Autodesk Inventor part; units mm, degrees
ref_plane "Arbeitsebene1" through (0, 0, 1.46) normal (0, 0, -1) x (-1, 0, 0)
ref_plane "Arbeitsebene2" through (-0.6, -3.21, 0) normal (0, -1, 0) x (1, 0, 0)
ref_plane "YZ Plane" through (0, 0, 0) normal (1, 0, 0) x (0, 1, 0)
sketch "Skizze2" plane through (0, 0, 0) normal (0, 0, 1) x (1, 0, 0)
  line L0 (0, 0) -> (-0.6, 0)
  line L1 (-0.6, 0) -> (-0.6, 0.6)
  line L2 (-0.6, 0.6) -> (0, 0.6)
  line L3 (0, 0.6) -> (0, 0)
  dimension "d0" = 0.6
  dimension "d1" = 0.6
extrude "Extrusion1" add sketch "Skizze2" along normal blind 9.46
ref_plane "Arbeitsebene1" through (0, 0, 1.46) normal (0, 0, -1) x (-1, 0, 0)
sketch "Skizze3" plane through (0, 0, 1.46) normal (0, 0, -1) x (-1, 0, 0)
  line L0 (1.57, 1.57) -> (-0.97, 1.57)
  line L1 (-0.97, 1.57) -> (-0.97, -0.97)
  line L2 (-0.97, -0.97) -> (1.57, -0.97)
  line L3 (1.57, -0.97) -> (1.57, 1.57)
  line L4 (0.6, 0) -> (0.6, 0.6)
  line L5 (0, 0.6) -> (0.6, 0.6)
  point P0 (0, 0)
  dimension "d5" = 2.54
  dimension "d6" = 2.54
  dimension "d7" = 0.97
  dimension "d8" = 0.97
extrude "Extrusion2" add sketch "Skizze3" against normal blind 2.5
chamfer "Fase1" distance 0.25 angle 45 4 edges at (0.97, -0.97, 2.71) (-1.57, -0.97, 2.71) (-1.57, 1.57, 2.71) (0.97, 1.57, 2.71)
sketch "Skizze8" plane through (-0.6, 0, 0) normal (0, -1, 0) x (1, 0, 0)
  line L0 (0, 0) -> (0.6, 0)
  line L1 (0, 0) -> (0, 1.46)
  line L2 (0.6, 0) -> (0, 0)
  line L3 (0, 0) -> (0, 0.6)
  line L4 (0, 0.6) -> (0.6, 0.6)
  line L5 (0.6, 0.6) -> (0.6, 0)
  dimension "d33" = 0.6
extrude "Extrusion6" add sketch "Skizze8" along normal blind 3.46
chamfer "Fase3" distance 0.15 angle 45 8 edges at (-0.6, 0.3, 9.46) (-0.3, 0, 9.46) (0, 0.3, 9.46) (-0.3, 0.6, 9.46) (0, -3.46, 0.3) (-0.3, -3.46, 0.6) (-0.3, -3.46, 0) (-0.6, -3.46, 0.3)
ref_plane "Arbeitsebene2" through (-0.6, -3.21, 0) normal (0, -1, 0) x (1, 0, 0)
sketch "Skizze10" plane through (-0.6, -3.21, 0) normal (0, -1, 0) x (1, 0, 0)
  circle A0 centre (0.3, 0.3) radius 0.325
  line L0 (0, 0) -> (0.6, 0)
  line L1 (0, 0.6) -> (0, 0)
  dimension "d40" = 0.65
  dimension "d41" = 0.3
  dimension "d42" = 0.3
extrude "Extrusion7" add sketch "Skizze10" against normal blind 0.5 contours A0 L0 L1 | L1 A0 | A0 L0 picked at (0.1927, 0.3972)
fillet "Rundung3" radius 1.4 1 edges at (-0.3, 0.6, 0)
fillet "Rundung4" radius 0.8 1 edges at (-0.3, 0, 0.6)
properties part number "Stiftleiste_Male_90_1"
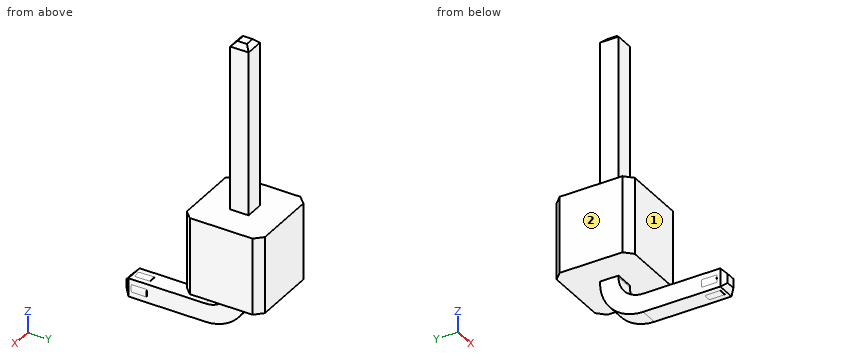
The model under review builds one solid part; all positions refer to its coordinate system, in mm. Face numbers are marked on the shaded views. A direction names the side the tool comes from. Round coordinates to 2 decimals unless told otherwise and drop trailing zeros. Order: outer loops, then holes, each group sorted by start corner. A loop starts at its lowest first (then second) coordinate and runs counter-clockwise, first axis right, second up. Notation, with made-up numbers: (8.25, 13.25) - (66.25, 13.25) arc R19 cw to (66.25, 30.25) - close; hole circle Ø9 at (64.5, 9.25). An arc over 180 degrees is marked (long way). Answer in a Markdown table with one row per item.
(1) For line 1 (Y direction, x = -0.45, z = 5.75); line 2 (Y direction, x = -0.4, z = 3.25); line 3 (Z direction, x = -0.05, y = 1.1), list the stretches that pass through material, from the lowest coordinate up. Write a range as from..to.
Result set:
| item | result |
|---|---|
| line 1 | y = 0..0.6 |
| line 2 | y = -0.97..1.57 |
| line 3 | z = 1.46..3.96 |
(2) Machinability: for the marked faces 1 and 2, which of the approach directions +Z, -Z, +X, -X, +Y, -Y give a long, thin tool a straight path to every point of the face, cutting with its end or side? Answer none if there is none.
Result set:
| item | result |
|---|---|
| face 1 | +Z, +X, -X, -Y |
| face 2 | +Z, -Z, -X, +Y, -Y |
(3) Take a section at D-D on x = 0.85. Write out the cut boundary in (y, z), plus the area to 3 significant figures.
Result set:
| item | result |
|---|---|
| outline | (-0.84, 1.46) - (1.44, 1.46) - (1.44, 3.96) - (-0.84, 3.96) - close |
| area | 5.70 mm2 |
(4) Clearance check with flat-ended pins moving along their axes: P1, Ø1.2, axis at y = -2, z = 0.5, coming from the +X side; P2, Ø1.5, axis at y = 1, z = 5, coming from the -X side; P3, Ø0.5, axis at x = -0.5, z = 5.5, coming from the -Y side. State where each tip first meets the part, or that it passes through.
Result set:
| item | result |
|---|---|
| P1 | stops at x = 0 |
| P2 | stops at x = -0.6 |
| P3 | stops at y = 0 |
(5) Take a section at B-B on z = 1.75. Write out the cut boundary in (x, y), plus the area to 3 significant figures.
Result set:
| item | result |
|---|---|
| outline | (-1.57, -0.72) - (-1.32, -0.97) - (0.72, -0.97) - (0.97, -0.72) - (0.97, 1.32) - (0.72, 1.57) - (-1.32, 1.57) - (-1.57, 1.32) - close |
| area | 6.33 mm2 |
(6) Take a section at C-C on y = -0.3. Write out the cut boundary in (x, z), plus the area to 3 significant figures.
Result set:
| item | result |
|---|---|
| outline | (-1.57, 1.46) - (0.97, 1.46) - (0.97, 3.96) - (-1.57, 3.96) - close; (-0.6, 0.09) - (0, 0.09) - (0, 0.78) - (-0.6, 0.78) - close |
| area | 6.76 mm2 |
(7) Take a section at A-A on y = -2.85. Write out the cut boundary in (x, z) (3 decimals).
Result set:
| item | result |
|---|---|
| outline | (-0.6, 0) - (-0.425, 0) arc R0.325 ccw to (-0.175, 0) - (0, 0) - (0, 0.175) arc R0.325 ccw to (0, 0.425) - (0, 0.6) - (-0.175, 0.6) arc R0.325 ccw to (-0.425, 0.6) - (-0.6, 0.6) - (-0.6, 0.425) arc R0.325 ccw to (-0.6, 0.175) - close |
